```python
from build123d import *

# Parameters (mm, degrees)
SKETCH1_W           = 15.5
SKETCH1_H           = 19.5
SKETCH1_W_2         = 9.9
SKETCH1_H_2         = 13.9
BOSS_EXTRUDE1_DEPTH = 4.05
SKETCH2_W           = 19.5
SKETCH2_H           = 9
SKETCH2_R           = 1.5
BOSS_EXTRUDE2_DEPTH = 2.8
CHAMFER1_SIZE       = 2.5
FILLET1_R           = 2
FILLET2_R           = 0.5
CHAMFER2_SIZE       = 0.5


with BuildPart() as part:
    # Sketch1 → Boss-Extrude1 (new body, symmetric)
    with BuildSketch(Plane(origin=(0, 0, 0), x_dir=(1, 0, 0), z_dir=(0, 1, 0))):
        Rectangle(SKETCH1_W, SKETCH1_H)
        Rectangle(SKETCH1_W_2, SKETCH1_H_2, mode=Mode.SUBTRACT)
    extrude(amount=BOSS_EXTRUDE1_DEPTH, both=True)

    # Sketch2 → Boss-Extrude2 (add)
    with BuildSketch(Plane.ZY.offset(7.75)):
        with Locations((0, -8.55)):
            Rectangle(SKETCH2_W, SKETCH2_H)
        with Locations((-5.25, -8.55)):
            Circle(SKETCH2_R, mode=Mode.SUBTRACT)
        with Locations((5.25, -8.55)):
            Circle(SKETCH2_R, mode=Mode.SUBTRACT)
    extrude(amount=-BOSS_EXTRUDE2_DEPTH)

    # Chamfer1
    chamfer1_edges = [part.edges().sort_by_distance(p)[0] for p in [
        (-4.95, -4.05, -8.35),
        (-4.95, -4.05, 8.35),
    ]]
    chamfer(chamfer1_edges, length=CHAMFER1_SIZE)

    # Fillet1
    fillet1_edges = [part.edges().sort_by_distance(p)[0] for p in [
        (-7.75, -4.5, -9.75),
        (7.75, 0, -9.75),
        (7.75, 0, 9.75),
        (-7.75, -4.5, 9.75),
    ]]
    fillet(fillet1_edges, radius=FILLET1_R)

    # Fillet2
    fillet2_edges = [part.edges().sort_by_distance(p)[0] for p in [
        (4.95, -4.05, 0),
        (1.25, -4.05, -6.95),
        (-4.95, 4.05, 0),
        (0, 4.05, 6.95),
        (4.95, 4.05, 0),
        (0, 4.05, -6.95),
        (-5.35, -13.05, -9.75),
        (-4.95, -9.8, 9.75),
        (-4.95, -13.05, 0),
        (-5.35, -13.05, 9.75),
        (1.65, -4.05, 9.75),
        (1.25, -4.05, 6.95),
        (-2.45, -4.05, 8.35),
        (-2.45, -4.05, -8.35),
        (-4.95, -9.8, -9.75),
        (-3.7, -5.3, -9.75),
        (-3.7, -5.3, -6.95),
        (-3.7, -5.3, 6.95),
        (-3.7, -5.3, 9.75),
        (1.65, -4.05, -9.75),
        (0, 4.05, -9.75),
        (7.75, -4.05, 0),
        (7.164213562, -4.05, 9.164213562),
        (7.164213562, -4.05, -9.164213562),
        (7.75, 4.05, 0),
        (-7.75, 4.05, 0),
        (0, 4.05, 9.75),
        (-7.164213562, 4.05, 9.164213562),
        (-7.164213562, 4.05, -9.164213562),
        (7.164213562, 4.05, 9.164213562),
        (7.164213562, 4.05, -9.164213562),
        (-7.75, -13.05, 0),
        (-7.164213562, -13.05, 9.164213562),
        (-7.164213562, -13.05, -9.164213562),
    ]]
    fillet(fillet2_edges, radius=FILLET2_R)

    # Chamfer2
    chamfer2_edges = [part.edges().sort_by_distance(p)[0] for p in [
        (-4.95, -8.55, 3.75),
        (-4.95, -8.55, -6.75),
    ]]
    chamfer(chamfer2_edges, length=CHAMFER2_SIZE)


solid = part.part
```
Read the model definition and answer for the solid it produces. Units are mm, in the model's axes. A direction names the side the tool comes from. Give positions to 0.01 mm unless a question says otherwise; leave off trailing zeros. Order: outer loops, then holes, each group sorted by start corner. A loop starts at its lowest first (then second) coordinate and runs counter-clockwise, first axis right, second up.
(1) Find section C-C (x = 4.5). Give the vertices of the cut face in (y, z).
(2) Find section D-D (z = -5.25). Give the vertices of the cut face in (x, y), plus the area to 3 significant figures.
(3) Straight lines are drawn through the part: L1, parallel to Y at x = -6.15, z = 5.25; L2, parallel to Z at x = 4.5, y = -1; L3, parallel to X at y = -3, z = -1. For each, find the intervals that lie inside material, in ascending order.
(4) For a pull along Y with two mould halves and no side action, classify faces 4 (the cylindrical face through (-6.616, -10.014, 4.925)), 5 (the flat face through (7.75, 0, 0)), 6 (the cylindrical face through (-4, -5.4, 9.6)) as released by +Y, released by -Y, zero draft, split by the parting line, or undercut.
(5) Find section B-B (y = -8.55). Give the vertices of the cut face in (x, z).
(6) For faces 1 (the flat face through (4.95, 0, 0)), 2 (the flat face through (-6, -13.05, 0)), 3 (the flat face through (6, -4.05, 0)), determine the directions among +Z, -Z, +X, -X, +Y, -Y from which every point of the face is accessible in a straight line to the end or side of a thin tool.
(7) Find section A-A (z = -1.25). Give the vertices of the cut face in (x, y).
(8) Given pin 1 (7.5 mm diameter, centred on x = 2, z = -3, fed in from -Y), flat-ended and moving along its own axis, determine where the tip first touches the part or whether it passes through.
Result sheet:
1. outline: (-4.05, -9.25) arc R0.5 ccw to (-3.55, -9.75) - (3.55, -9.75) arc R0.5 ccw to (4.05, -9.25) - (4.05, -7.45) arc R0.5 ccw to (3.55, -6.95) - (-3.55, -6.95) arc R0.5 ccw to (-4.05, -7.45) - close; (-4.05, 7.45) arc R0.5 ccw to (-3.55, 6.95) - (3.55, 6.95) arc R0.5 ccw to (4.05, 7.45) - (4.05, 9.25) arc R0.5 ccw to (3.55, 9.75) - (-3.55, 9.75) arc R0.5 ccw to (-4.05, 9.25) - close
2. outline: (-7.75, -12.55) arc R0.5 ccw to (-7.25, -13.05) - (-5.45, -13.05) arc R0.5 ccw to (-4.95, -12.55) - (-4.95, -10.55) - (-5.45, -10.05) - (-7.75, -10.05) - close; (-7.75, -7.05) - (-5.45, -7.05) - (-4.95, -6.55) - (-4.95, 3.55) arc R0.5 ccw to (-5.45, 4.05) - (-7.25, 4.05) arc R0.5 ccw to (-7.75, 3.55) - close; (4.95, -3.55) arc R0.5 ccw to (5.45, -4.05) - (7.25, -4.05) arc R0.5 ccw to (7.75, -3.55) - (7.75, 3.55) arc R0.5 ccw to (7.25, 4.05) - (5.45, 4.05) arc R0.5 ccw to (4.95, 3.55) - close
2. area: 61.5 mm2
3. L1: y = -13.05 to -10.05, -7.05 to 4.05
3. L2: z = -9.75 to -6.95, 6.95 to 9.75
3. L3: x = -7.75 to -4.95, 4.95 to 7.75
4. face 4: undercut
4. face 5: zero draft
4. face 6: released by -Y
5. outline: (-7.75, -7.75) arc R2 ccw to (-5.75, -9.75) - (-5.45, -9.75) arc R0.5 ccw to (-4.95, -9.25) - (-4.95, -7.25) - (-5.45, -6.75) - (-7.75, -6.75) - close; (-7.75, -3.75) - (-5.45, -3.75) - (-4.95, -3.25) - (-4.95, 3.25) - (-5.45, 3.75) - (-7.75, 3.75) - close; (-7.75, 6.75) - (-5.45, 6.75) - (-4.95, 7.25) - (-4.95, 9.25) arc R0.5 ccw to (-5.45, 9.75) - (-5.75, 9.75) arc R2 ccw to (-7.75, 7.75) - close
6. face 1: +Y, -Y
6. face 2: +Z, -Z, +X, -X, -Y
6. face 3: +Z, -Z, +X, -Y
7. outline: (-7.75, -12.55) arc R0.5 ccw to (-7.25, -13.05) - (-5.45, -13.05) arc R0.5 ccw to (-4.95, -12.55) - (-4.95, 3.55) arc R0.5 ccw to (-5.45, 4.05) - (-7.25, 4.05) arc R0.5 ccw to (-7.75, 3.55) - close; (4.95, -3.55) arc R0.5 ccw to (5.45, -4.05) - (7.25, -4.05) arc R0.5 ccw to (7.75, -3.55) - (7.75, 3.55) arc R0.5 ccw to (7.25, 4.05) - (5.45, 4.05) arc R0.5 ccw to (4.95, 3.55) - close
8. pin 1: stops at y = -4.05
